For this review, take the finished solid that the model builds, in its own axes (mm). A direction names the side the tool comes from. Give positions to 0.01 mm unless a question says otherwise; leave off trailing zeros. Loops run counter-clockwise (first coordinate to the right, second up) from the corner with the lowest first, then second, coordinate; pieces in that order, holes last. Notation, with made-up numbers: (-23, 22) - (-10, 22) arc R10 cw to (-10, 34) - close; hole circle Ø11 at (2, 25.25). An arc over 180 degrees is marked (long way). Answer as CSV lines item,"result".
from build123d import *

# Parameters (mm, degrees)
F0_R     = 2.5
F1_DEPTH = 4
F2_DEPTH = 3.5
F3_R     = 1.5
F4_DEPTH = 30
F5_R     = 0.2


with BuildPart() as f1:
    # F0 (on Top) → F1 (new body)
    with BuildSketch(Plane.XY):
        Circle(F0_R)
        Polygon((-1.3528307096, 1.0815956135), (0.2602739232, 1.7123835683), (1.6131046327, 0.6307879547), (1.3528307096, -1.0815956135), (-0.2602739232, -1.7123835683), (-1.6131046327, -0.6307879547), align=None, mode=Mode.SUBTRACT)
        Polygon((1.6131046327, 0.6307879547), (0.2602739232, 1.7123835683), (-1.3528307096, 1.0815956135), (-1.6131046327, -0.6307879547), (-0.2602739232, -1.7123835683), (1.3528307096, -1.0815956135), align=None)
    extrude(amount=F1_DEPTH)

    # F0 (on Top) → F2 (cut)
    with BuildSketch(Plane.XY):
        Polygon((1.6131046327, 0.6307879547), (0.2602739232, 1.7123835683), (-1.3528307096, 1.0815956135), (-1.6131046327, -0.6307879547), (-0.2602739232, -1.7123835683), (1.3528307096, -1.0815956135), align=None)
    extrude(amount=F2_DEPTH, mode=Mode.SUBTRACT)

    # F3 (on face) → F4 (join)
    with BuildSketch(Plane.XY.offset(4)):
        Circle(F3_R)
    extrude(amount=F4_DEPTH)

    # F5
    f5_edges = [f1.edges().sort_by_distance(p)[0] for p in [
        (-1.5, 0, 4),
        (-1.5, 0, 34),
        (2.5, 0, 2),
        (-2.5, 0, 0),
        (-2.5, 0, 4),
        (-0.546278, 1.39699, 0),
        (0.546278, -1.39699, 3.5),
        (1.482968, -0.225404, 3.5),
        (0.936689, 1.171586, 3.5),
        (-0.546278, 1.39699, 3.5),
        (-1.482968, 0.225404, 3.5),
        (-0.936689, -1.171586, 3.5),
        (0.546278, -1.39699, 0),
        (-0.936689, -1.171586, 0),
        (-1.482968, 0.225404, 0),
        (0.936689, 1.171586, 0),
        (1.482968, -0.225404, 0),
    ]]
    fillet(f5_edges, radius=F5_R)


solid = f1.part
1) Draft analysis for pull direction X (two halves, no side actions). For faces 1 (the cylindrical face through (-0.54, -2.44, 1.97)), 2 (the flat face through (0, 0, 3.5)), 3 (the flat face through (0, -2, 4)), state which applies: pulls with the +X half, pulls with the -X half, needs draft (parallel to the pull), parting line crosses it, or undercut.
From the geometry:
face 1,"parting line crosses it"
face 2,"undercut"
face 3,"needs draft"
2) Machinability: for faces 4 (the flat face through (0, 0, 34)), 5 (the flat face through (-0.535, 1.401, 1.728)), 6 (the cylindrical face through (-1.5, 0.07, 18.79)), which of the approach directions +Z, -Z, +X, -X, +Y, -Y give a long, thin tool a straight path to every point of the face, cutting with its end or side? Answer none if there is none.
From the geometry:
face 4,"+Z, +X, -X, +Y, -Y"
face 5,"-Z"
face 6,"+Z"
3) Consider section A-A on z = 21.5. Write out the cut boundary in (x, y).
From the geometry:
outline,"circle Ø3 at (0, 0)"
4) Insertion check: P1, Ø1, axis at y = 0.5, z = 25, coming from the +X side; P2, Ø1.4, axis at x = -0.5, y = 0, coming from the -Z side; P3, Ø2, axis at x = 1, z = 12, coming from the +Y side. Each pin has a flat end and moves straight along its axis. Give the tip position at first contact, or say it passes through.
From the geometry:
P1,"stops at x = 1.5"
P2,"stops at z = 3.5"
P3,"stops at y = 1.5"
5) Wall thickness on line 1 (Z direction, x = -0.85, y = 2); line 2 (Y direction, x = -0.75, z = 27.5); line 3 (Y direction, x = 0.65, z = 28.5): over which ranges is each line inside the solid? List them lowest first. Write a range as from..to.
From the geometry:
line 1,"z = 0..4"
line 2,"y = -1.3..1.3"
line 3,"y = -1.35..1.35"
